```python
from build123d import *

# Parameters (mm, degrees)
F0_W     = 127
F0_H     = 228.6
F1_DEPTH = 50.8
F2_SIZE  = 12.7
F3_SIZE  = 6.35
F4_W     = 82.55
F4_H     = 69.85
F5_DEPTH = 25.4


with BuildPart() as f1:
    # F0 (on Front) → F1 (new body, symmetric)
    with BuildSketch(Plane.XZ):
        Rectangle(F0_W, F0_H)
    extrude(amount=F1_DEPTH, both=True)

    # F2
    f2_edges = [f1.edges().sort_by_distance(p)[0] for p in [
        (-63.5, 0, 114.3),
        (63.5, 0, 114.3),
        (63.5, 0, -114.3),
        (-63.5, 0, -114.3),
    ]]
    chamfer(f2_edges, length=F2_SIZE)

    # F3
    f3_edges = [f1.edges().sort_by_distance(p)[0] for p in [
        (0, -50.8, -114.3),
        (-57.15, -50.8, -107.95),
        (57.15, -50.8, -107.95),
        (-63.5, -50.8, 0),
        (63.5, -50.8, 0),
        (-57.15, -50.8, 107.95),
        (57.15, -50.8, 107.95),
        (0, -50.8, 114.3),
        (0, 50.8, -114.3),
        (-57.15, 50.8, -107.95),
        (57.15, 50.8, -107.95),
        (-63.5, 50.8, 0),
        (63.5, 50.8, 0),
        (-57.15, 50.8, 107.95),
        (57.15, 50.8, 107.95),
        (0, 50.8, 114.3),
    ]]
    chamfer(f3_edges, length=F3_SIZE)

    # F4 (on face) → F5 (cut)
    with BuildSketch(Plane(origin=(0, 0, -114.3), x_dir=(1, 0, 0), z_dir=(0, 0, -1))):
        Rectangle(F4_W, F4_H)
    extrude(amount=-F5_DEPTH, mode=Mode.SUBTRACT)


solid = f1.part
```
Check sheet for the modelled part. Datum: model origin and axes. Units: mm. A direction names the side the tool comes from. Give positions to 0.01 mm unless a question says otherwise; leave off trailing zeros. Order: outer loops, then holes, each group sorted by start corner. A loop starts at its lowest first (then second) coordinate and runs counter-clockwise, first axis right, second up. Notation, with made-up numbers: (-27, 36) -> (18, 36) arc R11 ccw to (18, 46) -> close; hole circle Ø8 at (89, 87.5). An arc over 180 degrees is marked (long way). Return JSON: item names as keys, results as strings.
1. Set-up check for faces 1 (the flat face through (41.275, 0, -102)), 2 (the flat face through (-1, -50.8, 2)): record each of +Z, -Z, +X, -X, +Y, -Y from which the full face is reachable in a straight line by a thin tool's end or side.
From the geometry:
{"face 1": "-Z", "face 2": "+Z, -Z, +X, -X, -Y"}
2. Cross-section at A-A, the plane x = -29. Record the cut outline in (y, z) (3 decimals), plus the area to 3 significant figures.
From the geometry:
{"outline": "(-50.8, -107.95) -> (-44.45, -114.3) -> (-34.925, -114.3) -> (-34.925, -88.9) -> (34.925, -88.9) -> (34.925, -114.3) -> (44.45, -114.3) -> (50.8, -107.95) -> (50.8, 107.95) -> (44.45, 114.3) -> (-44.45, 114.3) -> (-50.8, 107.95) -> close", "area": "21,400 mm^2"}
3. Go/stop test with a flat-tipped pin: P1, Ø4, axis at x = 6, y = 22.5, coming from the -Z side. Record where the tip stops, or that it passes through.
From the geometry:
{"P1": "z = -88.9"}
4. Material ranges on probe 1 along X at (y, z) = (32.5, -91.5) (3 decimals); probe 2 along Z at (x, y) = (3, -5.5); probe 3 along X at (y, z) = (-44.5, -13), recorded low to high. Write a range as [from, to].
From the geometry:
{"probe 1": "[-63.5, -41.275], [41.275, 63.5]", "probe 2": "[-88.9, 114.3]", "probe 3": "[-63.45, 63.45]"}
5. Cross-section at B-B, the plane y = -8. Record the cut outline in (x, z) (3 decimals), plus the area to 3 significant figures.
From the geometry:
{"outline": "(-63.5, -101.6) -> (-50.8, -114.3) -> (-41.275, -114.3) -> (-41.275, -88.9) -> (41.275, -88.9) -> (41.275, -114.3) -> (50.8, -114.3) -> (63.5, -101.6) -> (63.5, 101.6) -> (50.8, 114.3) -> (-50.8, 114.3) -> (-63.5, 101.6) -> close", "area": "26,600 mm^2"}
6. Cross-section at C-C, the plane z = -94. Record the cut outline in (x, y) (3 decimals), plus the area to 3 significant figures.
From the geometry:
{"outline": "(-63.5, -44.45) -> (-57.15, -50.8) -> (57.15, -50.8) -> (63.5, -44.45) -> (63.5, 44.45) -> (57.15, 50.8) -> (-57.15, 50.8) -> (-63.5, 44.45) -> close; hole (-41.275, -34.925) -> (41.275, -34.925) -> (41.275, 34.925) -> (-41.275, 34.925) -> close", "area": "7,060 mm^2"}
7. Mould release check, pull along Y, two halves, no side actions. Record for faces 3 (the flat face through (-1, -34.925, -102)), 4 (the flat face through (-0.71, -47.58, 111.17)), 5 (the flat face through (55.025, 47.581, -105.647)), 6 (the flat face through (-1, 34.925, -102)): +Y half, -Y half, draft (parallel to the pull), parting line (faces both ways), or undercut.
From the geometry:
{"face 3": "undercut", "face 4": "-Y half", "face 5": "+Y half", "face 6": "undercut"}
